Verification items for this drawing (mm, ordinates from the low corner). A direction names the side the tool comes from. Coordinates: 2 decimals unless noted, no trailing zeros. Write each loop counter-clockwise with the first axis right and the second up, starting at its lowest first coordinate (ties: lowest second). Pieces come first, ordered by that corner, then holes. Notation, with made-up numbers: (37.25, 9.25) -> (83.25, 9.25) arc R24 cw to (83.25, 29.25) -> close; hole circle Ø3 at (-12, 55). An arc over 180 degrees is marked (long way). One line per question, with ' | ' between items.
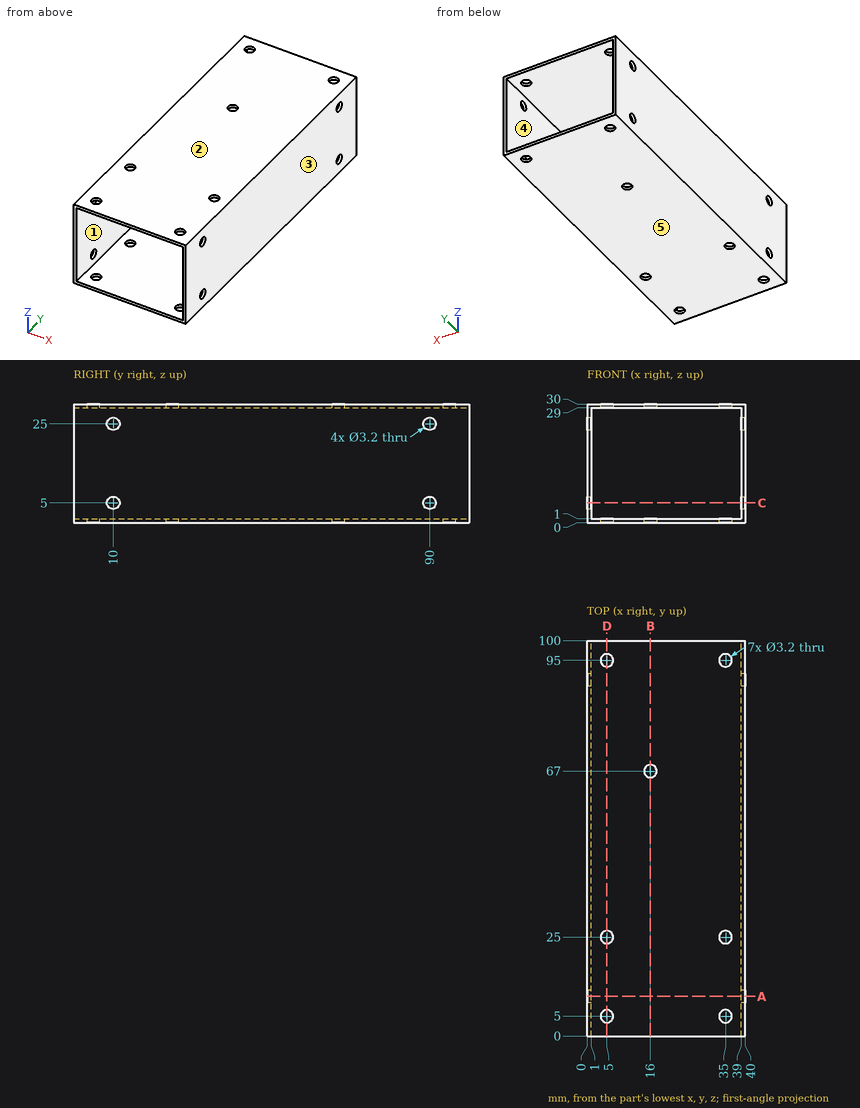
(1) Material ranges on line 1 (X direction, y = 95, z = 29.4); line 2 (Y direction, x = 5, z = 0.35); line 3 (X direction, y = 46, z = 5.75), recorded low to high.
Answers below:
line 1: x = 0 to 3.4, 6.6 to 33.4, 36.6 to 40 | line 2: y = 0 to 3.4, 6.6 to 23.4, 26.6 to 93.4, 96.6 to 100 | line 3: x = 0 to 1, 39 to 40
(2) Cross-section at D-D (x = 5). Count the separate pieces of the cut face and the enclosed holes in it, plus the area to 3 significant figures.
Answers below:
separate pieces: 8 | enclosed holes: 0 | area: 181 mm²
(3) Cross-section at A-A (y = 10). Record the cut outline in (x, z).
Answers below:
outline: (0, 0) -> (40, 0) -> (40, 3.4) -> (39, 3.4) -> (39, 1) -> (1, 1) -> (1, 3.4) -> (0, 3.4) -> close; (0, 6.6) -> (1, 6.6) -> (1, 23.4) -> (0, 23.4) -> close; (0, 26.6) -> (1, 26.6) -> (1, 29) -> (39, 29) -> (39, 26.6) -> (40, 26.6) -> (40, 30) -> (0, 30) -> close; (39, 6.6) -> (40, 6.6) -> (40, 23.4) -> (39, 23.4) -> close
(4) Tool access check on the marked faces 4 and 5. Record the directions out of +Z, -Z, +X, -X, +Y, -Y that give a thin tool (end or side, any length) a straight path to the whole face; none if there is none.
Answers below:
face 4: +Y, -Y | face 5: -Z, +X, -X, +Y, -Y
(5) Draft check along Z on the marked faces 1, 2 and 3. Enter one of: pulls with the +Z half, pulls with the -Z half, needs draft (parallel to the pull), parting line crosses it, or undercut.
Answers below:
face 1: undercut | face 2: pulls with the +Z half | face 3: needs draft
(6) Cross-section at B-B (x = 16). Record the cut outline in (y, z), plus the area to 3 significant figures.
Answers below:
outline: (0, 0) -> (65.4, 0) -> (65.4, 1) -> (0, 1) -> close; (0, 29) -> (65.4, 29) -> (65.4, 30) -> (0, 30) -> close; (68.6, 0) -> (100, 0) -> (100, 1) -> (68.6, 1) -> close; (68.6, 29) -> (100, 29) -> (100, 30) -> (68.6, 30) -> close | area: 194 mm²
(7) Cross-section at C-C (z = 5). Record the cut outline in (x, y), plus the area to 3 significant figures.
Answers below:
outline: (0, 0) -> (1, 0) -> (1, 8.4) -> (0, 8.4) -> close; (0, 11.6) -> (1, 11.6) -> (1, 88.4) -> (0, 88.4) -> close; (0, 91.6) -> (1, 91.6) -> (1, 100) -> (0, 100) -> close; (39, 0) -> (40, 0) -> (40, 8.4) -> (39, 8.4) -> close; (39, 11.6) -> (40, 11.6) -> (40, 88.4) -> (39, 88.4) -> close; (39, 91.6) -> (40, 91.6) -> (40, 100) -> (39, 100) -> close | area: 187 mm²
